Part model, mm, in its own coordinate system. A direction names the side the tool comes from. Coordinates: 2 decimals unless noted, no trailing zeros. Loops run counter-clockwise (first coordinate to the right, second up) from the corner with the lowest first, then second, coordinate; pieces in that order, holes last. Notation, with made-up numbers: M 62,63.25 L 72,63.25 A28 cw 72,93.25 Z; hole C 77,73.25 d3. An arc over 180 degrees is marked long. Use a Markdown table: item, result. Add a question column.
1) Wall check: probe 1 along Y at (x, z) = (457.2, -97); probe 2 along Z at (x, y) = (147, 116); probe 3 along Z at (x, y) = (786, -155). Give the ranges that are in metal, low to high. Write a range as from..to.
2) Band-saw the part on D-D (y = -204.5). List the corners of the cut face in (x, z), plus the area to 3 significant figures.
3) Pull direction X, two halves, no side cores. Call faces 4 (the cylindrical face through (-97.505, -3.556, -54.618)), 5 (the cylindrical face through (215.958, -84.065, 333.85)), 6 (the flat face through (366.63, -1.78, 484.56)): released by +X, released by -X, zero draft, split by the parting line, or undercut.
4) Tool access for faces 1 (the flat face through (644, -4, -63.5)), 2 (the cylindrical face through (339.81, 217.78, 457.35)), 3 (the flat face through (968, 63.5, -87)): list every direction of +Z, -Z, +X, -X, +Y, -Y with a clear straight run to the whole face (end or side of a thin tool).
5) Pin check, flat tips, straight feed: pin 1 Ø10 at (y, z) = (-31.5, 64.5) entering from -X; pin 2 Ø6 at (y, z) = (-171.5, 169) entering from +X; pin 3 Ø8 at (y, z) = (-2, 232.5) entering from +X. Stop position of each tip, or through.
6) Band-saw the part on B-B (y = 21). List the corners of the cut face in (x, z), plus the area to 3 significant figures.
7) Band-saw the part on C-C (y = 209). List the corners of the cut face in (x, z).
8) Band-saw the part on A-A (x = 457.2). List the corners of the cut face in (y, z), plus the area to 3 significant figures.
from build123d import *

# Parameters (mm, degrees)
F1_DEPTH = 254
F2_R     = 63.5
F3_DEPTH = 48.261
F4_R     = 38.1
F5_DEPTH = 49.6377001669
F6_R     = 127
F7_R     = 127


# Not quite as in the source:
# - a pattern or mirror of a feature is missing from the dataset's text; its kind, count and spacing are read off the source's solid


with BuildPart() as f1:
    # F0 (on Front) → F1 (new body, symmetric)
    with BuildSketch(Plane.XZ):
        with BuildLine():
            Line((1270, -63.5), (0, -63.5))
            ThreePointArc((0, -63.5), (-50.8447137485, -38.0403086717), (-60.9180663091, 17.9231469658))
            Line((-60.9180663091, 17.9231469658), (383.0492185975, 467.3498327088))
            Line((383.0492185975, 467.3498327088), (349.7351963182, 502.2669276563))
            Line((349.7351963182, 502.2669276563), (-96.9701293302, 55.5616020078))
            ThreePointArc((-96.9701293302, 55.5616020078), (-96.6950418594, -56.0389728653), (0, -111.76))
            Line((0, -111.76), (1270, -111.76))
            Line((1270, -111.76), (1270, -63.5))
        make_face()
    extrude(amount=F1_DEPTH, both=True)

    # F2 (on face) → F3 (cut, through all)
    with BuildSketch(Plane.XY.offset(-63.5)):
        with BuildLine():
            ThreePointArc((1155.7, -63.5), (1200.6012806053, -44.9012806053), (1219.2, 0))
            ThreePointArc((1219.2, 0), (1200.6012806053, 44.9012806053), (1155.7, 63.5))
            ThreePointArc((1155.7, 63.5), (1092.2, 0), (1155.7, -63.5))
        make_face()
        with BuildLine():
            ThreePointArc((1155.7, -63.5), (1092.2, 0), (1155.7, 63.5))
            Line((1155.7, 63.5), (774.7, 63.5))
            ThreePointArc((774.7, 63.5), (819.6012806053, 44.9012806053), (838.2, 0))
            ThreePointArc((838.2, 0), (819.6012806053, -44.9012806053), (774.7, -63.5))
            Line((774.7, -63.5), (1155.7, -63.5))
        make_face()
        with BuildLine():
            ThreePointArc((838.2, 0), (819.6012806053, 44.9012806053), (774.7, 63.5))
            ThreePointArc((774.7, 63.5), (711.2, 0), (774.7, -63.5))
            ThreePointArc((774.7, -63.5), (819.6012806053, -44.9012806053), (838.2, 0))
        make_face()
        with Locations((457.2, 0)):
            Circle(F2_R)
    extrude(amount=-F3_DEPTH, mode=Mode.SUBTRACT)

    # F4 (on face) → F5 (cut, through all)
    with BuildSketch(Plane(origin=(-76.265865669, 0, 76.265865669), x_dir=(0, -1, 0), z_dir=(-0.7071067812, 0, 0.7071067812))):
        with Locations((114.3, 411.9564794477)):
            Circle(F4_R)
    f5 = extrude(amount=-F5_DEPTH, mode=Mode.SUBTRACT)

    # F5_copies: F5 across plane
    add(f5.mirror(Plane.ZX.offset(-1e-06)), mode=Mode.SUBTRACT)

    # F6
    f6_edges = [f1.edges().sort_by_distance(p)[0] for p in [
        (366.392207, 254, 484.80838),
        (366.392207, -254, 484.80838),
    ]]
    fillet(f6_edges, radius=F6_R)

    # F7
    f7_edges = [f1.edges().sort_by_distance(p)[0] for p in [
        (1270, 254, -87.63),
        (1270, -254, -87.63),
    ]]
    fillet(f7_edges, radius=F7_R)


solid = f1.part
Entries:
| question | item | result |
|---|---|---|
| 1 | probe 1 | -254..-63.5, 63.5..254 |
| 1 | probe 2 | -111.76..-63.5, 228.4..299.53 |
| 1 | probe 3 | -111.76..-63.5 |
| 2 | outline | M -96.97,55.56 A111.76 ccw 0,-111.76 L 1243.61,-111.76 L 1243.61,-63.5 L 0,-63.5 A63.5 cw -60.92,17.92 L 364.5,448.57 L 331.07,483.6 Z |
| 2 | area | 98,900 mm2 |
| 3 | face 4 | released by -X |
| 3 | face 5 | undercut |
| 3 | face 6 | released by +X |
| 4 | face 1 | +X, +Y, -Y |
| 4 | face 2 | +Z, +X, +Y |
| 4 | face 3 | +Z, -Z |
| 5 | pin 1 | x = -93.03 |
| 5 | pin 2 | x = 91.29 |
| 5 | pin 3 | x = 155 |
| 6 | outline | M -96.97,55.56 A111.76 ccw 0,-111.76 L 397.27,-111.76 L 397.27,-63.5 L 0,-63.5 A63.5 cw -60.92,17.92 L 383.05,467.35 L 349.74,502.27 Z; M 517.13,-111.76 L 714.77,-111.76 L 714.77,-63.5 L 517.13,-63.5 Z; M 1215.63,-111.76 L 1270,-111.76 L 1270,-63.5 L 1215.63,-63.5 Z |
| 6 | area | 71,500 mm2 |
| 7 | outline | M -96.97,55.56 A111.76 ccw 0,-111.76 L 1239.98,-111.76 L 1239.98,-63.5 L 0,-63.5 A63.5 cw -60.92,17.92 L 361.94,445.98 L 328.5,481.03 Z |
| 8 | outline | M -254,-111.76 L -63.5,-111.76 L -63.5,-63.5 L -254,-63.5 Z; M 63.5,-111.76 L 254,-111.76 L 254,-63.5 L 63.5,-63.5 Z |
| 8 | area | 18,400 mm2 |
